Autodesk Fusion 360 part; units mm, degrees
sketch "Sketch1" plane through (0, 0, 0) normal (0, 0, 1) x (1, 0, 0)
  circle A0 centre (0, 0) radius 6.55
  circle A1 centre (0, 0) radius 12.5
  dimension "d1" = 13.1
  dimension "d2" = 25
extrude "Extrude1" add sketch "Sketch1" along normal blind 6
sketch "Sketch2" plane through (0, 0, 0) normal (0, 1, 0) x (1, 0, 0)
  line L0 (-12.5, -6) -> (12.5, -6)
  line L1 (-12.5, 0) -> (12.5, 0)
  line L2 (12.5, 0) -> (9.5, -3)
  line L3 (9.5, -3) -> (12.5, -6)
  line L4 (12.5, -6) -> (12.5, 0)
  dimension "d5" = 45
  dimension "d6" = 45
revolve "Revolve1" cut sketch "Sketch2" angle 360 about axis through (0, 0, 1.75) along (0, 0, 1)
fillet "Fillet1" radius 0.5 2 edges at (-11.6541, -4.5202, 0) (-11.6541, -4.5202, 6)
Input: part model. Units: mm. Frame: model coordinates. A direction names the side the tool comes from. Give positions to 0.01 mm unless a question says otherwise; leave off trailing zeros. Order: outer loops, then holes, each group sorted by start corner. A loop starts at its lowest first (then second) coordinate and runs counter-clockwise, first axis right, second up. Notation, with made-up numbers: (75.5, -12.75) - (86.5, -12.75) arc R18 cw to (86.5, -4.75) - close; hole circle Ø5 at (89, 67.5). An arc over 180 degrees is marked (long way). Write each question's results on one line, items separated by ' | '.
Item 1: Contact query for flat-ended pins moving along their axis: pin 1 Ø1.5 at (x, z) = (5.5, 2) entering from +Y; pin 2 Ø12 at (x, y) = (0, 0) entering from +Z; pin 3 Ø1.5 at (y, z) = (-1.5, 0.5) entering from +X. Output: stop coordinate, or through.
A:
pin 1: stops at y = 9.91 | pin 2: passes through | pin 3: stops at x = 11.77
Item 2: Material intervals for line 1 along Z through (x, y) = (7.75, -7.5); line 2 along Y through (x, z) = (1, 5.75); line 3 along Y through (x, z) = (-4.75, 0.75), sorted ascending.
A:
line 1: z = 0 to 1.72, 4.28 to 6 | line 2: y = -11.68 to -6.47, 6.47 to 11.68 | line 3: y = -10.72 to -4.51, 4.51 to 10.72
Item 3: Section A-A (x = 0). Return loops of the section in (y, z).
A:
outline: (-11.65, 0.85) arc R0.5 ccw to (-11.29, 0) - (-6.55, 0) - (-6.55, 6) - (-11.29, 6) arc R0.5 ccw to (-11.65, 5.15) - (-9.5, 3) - close; (6.55, 0) - (11.29, 0) arc R0.5 ccw to (11.65, 0.85) - (9.5, 3) - (11.65, 5.15) arc R0.5 ccw to (11.29, 6) - (6.55, 6) - close
Item 4: Section D-D (z = 4.5). Return loops of the section in (x, y), and give its area (3 significant figures).
A:
outline: circle Ø22 at (0, 0); hole circle Ø13.1 at (0, 0) | area: 245 mm^2
Item 5: Access query for faces 4 (the cylindrical face through (-0.853, -6.494, 2.958)), 5 (the conical face through (-2.089, 9.405, 2.866)). Directions: +Z, -Z, +X, -X, +Y, -Y. A direction counts if a zero-diameter tool reaches every point of the face in a straight line with its end or side. Return the directions, or none.
A:
face 4: +Z, -Z | face 5: none
Item 6: Draft query along Z for faces 1 (the flat face through (5, -5, 6)), 2 (the flat face through (5, -5, 0)), 3 (the conical face through (-2.089, -9.405, 3.134)). Return one class per face: released by +Z, released by -Z, zero draft, split by the parting line, or undercut.
A:
face 1: released by +Z | face 2: released by -Z | face 3: undercut
Item 7: Section C-C (z = 0.5). Return loops of the section in (x, y).
A:
outline: circle Ø23.59 at (0, 0); hole circle Ø13.1 at (0, 0)
